from build123d import *
from build123d.topology import SkipClean

# Parameters (mm, degrees)
CIRPATTERN2_COUNT  = 6
SKETCH8_R          = 2.286
CUT_EXTRUDE1_DEPTH = 117.853803532


with BuildPart() as part:
    # Sketch3 → Revolve1 (revolve)
    with BuildSketch(Plane(origin=(0, 0, 0), x_dir=(0, 0, -1), z_dir=(1, 0, 0)), mode=Mode.PRIVATE) as revolve1_sk:
        with BuildLine():
            Line((0, 29.21), (0, 58.42))
            ThreePointArc((0, 58.42), (0.371974388, 59.318025612), (1.27, 59.69))
            Line((1.27, 59.69), (10.069743879, 59.69))
            ThreePointArc((10.069743879, 59.69), (12.499783674, 60.173364969), (14.559871939, 61.549871939))
            Line((14.559871939, 61.549871939), (21.000128061, 67.990128061))
            ThreePointArc((21.000128061, 67.990128061), (23.060216326, 69.366635031), (25.490256121, 69.85))
            Line((25.490256121, 69.85), (40.64, 69.85))
            Line((40.64, 69.85), (40.64, 77.47))
            Line((40.64, 77.47), (43.18, 77.47))
            Line((43.18, 77.47), (43.18, 67.31))
            Line((43.18, 67.31), (24.1935, 67.31))
            Line((24.1935, 67.31), (14.0335, 57.15))
            Line((14.0335, 57.15), (8.4455, 57.15))
            Line((8.4455, 57.15), (8.4455, 54.61))
            Line((8.4455, 54.61), (4.445, 54.61))
            ThreePointArc((4.445, 54.61), (3.546974388, 54.238025612), (3.175, 53.34))
            Line((3.175, 53.34), (3.175, 29.21))
            Line((3.175, 29.21), (0, 29.21))
        make_face()
    revolve(revolve1_sk.sketch.rotate(Axis((0, 0, 0), (0, 0, -1)), 90), axis=Axis((0, 0, 0), (0, 0, -1)))

    # Sketch7 → CSK for M4 Countersunk Flat Head Screw2 (revolve, cut)
    with BuildSketch(Plane(origin=(0, 35, -3.175), x_dir=(0, 1, 0), z_dir=(1, 0, 0))):
        Polygon((0, 0), (0, 4.526936393), (2.25, 3.175), (2.25, 2.45), (4.7, 0), align=None)
    csk_for_m4_countersunk_flat_head_screw2 = revolve(axis=Axis((0, 35, -9.525), (0, 0, 1)), mode=Mode.SUBTRACT)

    # CirPattern2: CSK for M4 Countersunk Flat Head Screw2 ×6 about axis
    cirpattern2_axis = Axis((0, 0, 0), (0, 0, 1))
    for i in range(1, CIRPATTERN2_COUNT):
        add(csk_for_m4_countersunk_flat_head_screw2.rotate(cirpattern2_axis, i * 360 / CIRPATTERN2_COUNT), mode=Mode.SUBTRACT)

    # Sketch8 → Cut-Extrude1 (cut, through all)
    with SkipClean():  # the faces are left unmerged after this step: merging them gives an invalid solid
        with BuildSketch(Plane.XY.offset(-40.64)):
            with BuildLine():
                ThreePointArc((77.47, 0), (75.984990618, 15.095764333), (71.586894261, 29.612792338))
                ThreePointArc((71.586894261, 29.612792338), (72.045629184, 26.639866522), (71.084638604, 23.789388889))
                Line((71.084638604, 23.789388889), (68.920030414, 20.36953457))
                ThreePointArc((68.920030414, 20.36953457), (68.026910163, 18.04667064), (68.095090227, 15.558958417))
                ThreePointArc((68.095090227, 15.558958417), (69.409886012, 7.828807306), (69.85, 0))
                ThreePointArc((69.85, 0), (69.409886012, -7.828807306), (68.095090227, -15.558958417))
                ThreePointArc((68.095090227, -15.558958417), (68.026910163, -18.04667064), (68.920030414, -20.36953457))
                Line((68.920030414, -20.36953457), (71.084638604, -23.789388889))
                ThreePointArc((71.084638604, -23.789388889), (72.045629184, -26.639866522), (71.586894261, -29.612792338))
                ThreePointArc((71.586894261, -29.612792338), (75.984990618, -15.095764333), (77.47, 0))
            make_face()
            with BuildLine():
                ThreePointArc((10.148016689, -76.802465177), (38.735, -67.090988031), (61.438877572, -47.189672839))
                ThreePointArc((61.438877572, -47.189672839), (59.093615754, -49.073411844), (56.14453442, -49.666408405))
                Line((56.14453442, -49.666408405), (52.100549608, -49.501729883))
                ThreePointArc((52.100549608, -49.501729883), (49.642330309, -49.889697022), (47.521998359, -51.192598801))
                ThreePointArc((47.521998359, -51.192598801), (41.484889014, -56.196320907), (34.925, -60.491874454))
                ThreePointArc((34.925, -60.491874454), (27.924996998, -64.025128213), (20.573091868, -66.751557218))
                ThreePointArc((20.573091868, -66.751557218), (18.384579854, -67.936367662), (16.819480806, -69.871264453))
                Line((16.819480806, -69.871264453), (14.940104183, -73.455797294))
                ThreePointArc((14.940104183, -73.455797294), (12.952013431, -75.713278366), (10.148016689, -76.802465177))
            make_face()
            with BuildLine():
                ThreePointArc((-56.14453442, -49.666408405), (-59.093615754, -49.073411844), (-61.438877572, -47.189672839))
                ThreePointArc((-61.438877572, -47.189672839), (-38.735, -67.090988031), (-10.148016689, -76.802465177))
                ThreePointArc((-10.148016689, -76.802465177), (-12.952013431, -75.713278366), (-14.940104183, -73.455797294))
                Line((-14.940104183, -73.455797294), (-16.819480806, -69.871264453))
                ThreePointArc((-16.819480806, -69.871264453), (-18.384579854, -67.936367662), (-20.573091868, -66.751557218))
                ThreePointArc((-20.573091868, -66.751557218), (-27.924996998, -64.025128213), (-34.925, -60.491874454))
                ThreePointArc((-34.925, -60.491874454), (-41.484889014, -56.196320907), (-47.521998359, -51.192598801))
                ThreePointArc((-47.521998359, -51.192598801), (-49.642330309, -49.889697022), (-52.100549608, -49.501729883))
                Line((-52.100549608, -49.501729883), (-56.14453442, -49.666408405))
            make_face()
            with BuildLine():
                ThreePointArc((-71.084638604, 23.789388889), (-72.045629184, 26.639866522), (-71.586894261, 29.612792338))
                ThreePointArc((-71.586894261, 29.612792338), (-77.47, 0), (-71.586894261, -29.612792338))
                ThreePointArc((-71.586894261, -29.612792338), (-72.045629184, -26.639866522), (-71.084638604, -23.789388889))
                Line((-71.084638604, -23.789388889), (-68.920030414, -20.36953457))
                ThreePointArc((-68.920030414, -20.36953457), (-68.026910163, -18.04667064), (-68.095090227, -15.558958417))
                ThreePointArc((-68.095090227, -15.558958417), (-69.409886012, -7.828807306), (-69.85, 0))
                ThreePointArc((-69.85, 0), (-69.409886012, 7.828807306), (-68.095090227, 15.558958417))
                ThreePointArc((-68.095090227, 15.558958417), (-68.026910163, 18.04667064), (-68.920030414, 20.36953457))
                Line((-68.920030414, 20.36953457), (-71.084638604, 23.789388889))
            make_face()
            with BuildLine():
                ThreePointArc((-14.940104183, 73.455797294), (-12.952013431, 75.713278366), (-10.148016689, 76.802465177))
                ThreePointArc((-10.148016689, 76.802465177), (-38.735, 67.090988031), (-61.438877572, 47.189672839))
                ThreePointArc((-61.438877572, 47.189672839), (-59.093615754, 49.073411844), (-56.14453442, 49.666408405))
                Line((-56.14453442, 49.666408405), (-52.100549608, 49.501729883))
                ThreePointArc((-52.100549608, 49.501729883), (-49.642330309, 49.889697022), (-47.521998359, 51.192598801))
                ThreePointArc((-47.521998359, 51.192598801), (-41.484889014, 56.196320907), (-34.925, 60.491874454))
                ThreePointArc((-34.925, 60.491874454), (-27.924996998, 64.025128213), (-20.573091868, 66.751557218))
                ThreePointArc((-20.573091868, 66.751557218), (-18.384579854, 67.936367662), (-16.819480806, 69.871264453))
                Line((-16.819480806, 69.871264453), (-14.940104183, 73.455797294))
            make_face()
            with BuildLine():
                ThreePointArc((10.148016689, 76.802465177), (12.952013431, 75.713278366), (14.940104183, 73.455797294))
                Line((14.940104183, 73.455797294), (16.819480806, 69.871264453))
                ThreePointArc((16.819480806, 69.871264453), (18.384579854, 67.936367662), (20.573091868, 66.751557218))
                ThreePointArc((20.573091868, 66.751557218), (27.924996998, 64.025128213), (34.925, 60.491874454))
                ThreePointArc((34.925, 60.491874454), (41.484889014, 56.196320907), (47.521998359, 51.192598801))
                ThreePointArc((47.521998359, 51.192598801), (49.642330309, 49.889697022), (52.100549608, 49.501729883))
                Line((52.100549608, 49.501729883), (56.14453442, 49.666408405))
                ThreePointArc((56.14453442, 49.666408405), (59.093615754, 49.073411844), (61.438877572, 47.189672839))
                ThreePointArc((61.438877572, 47.189672839), (38.735, 67.090988031), (10.148016689, 76.802465177))
            make_face()
            with Locations((0, 73.025)):
                Circle(SKETCH8_R)
            with Locations((63.241505111, 36.5125)):
                Circle(SKETCH8_R)
            with Locations((-63.241505111, 36.5125)):
                Circle(SKETCH8_R)
            with Locations((-63.241505111, -36.5125)):
                Circle(SKETCH8_R)
            with Locations((63.241505111, -36.5125)):
                Circle(SKETCH8_R)
            with Locations((0, -73.025)):
                Circle(SKETCH8_R)
        extrude(amount=-CUT_EXTRUDE1_DEPTH, mode=Mode.SUBTRACT)


solid = part.part
Geometry check sheet. Reference: the model listing, model coordinates, mm. A direction names the side the tool comes from. Round coordinates to 2 decimals unless told otherwise and drop trailing zeros. Write each loop counter-clockwise with the first axis right and the second up, starting at its lowest first coordinate (ties: lowest second). Pieces come first, ordered by that corner, then holes. Notation, with made-up numbers: (85, 2.25) -> (111, 2.25) arc R12 ccw to (111, 11.25) -> close; hole circle Ø7 at (13, 69.25). An arc over 180 degrees is marked (long way). One line per item, written item: value. Start each with the question number.
(1) Access from +Z, -Z, +X, -X, +Y, -Y to the whole of each face (thin tool, end or side, straight path). Record for faces 4 (the cylindrical face through (67.162, -38.612, -41.928)), 5 (the flat face through (60.8, -36.1, -40.64)), 6 (the flat face through (23, 23, -3.175)), 7 (the flat face through (60.8, 35.9, -40.64)), 8 (the cylindrical face through (12.917, 75.738, -41.892)).
(2) Go/stop test with flat-tipped pins: pin 1 Ø3.5 at (x, y) = (-30.31, 17.5) entering from +Z; pin 2 Ø10 at (x, y) = (-43.5, 6.5) entering from -Z (3 decimals); pin 3 Ø5 at (x, z) = (37.5, -30.5) entering from +Y; pin 4 Ø2 at (x, y) = (-39.5, 56) entering from +Z. Record where each tip stops, or that it passes through.
(3) Scan lines: line 1 (X direction, y = -2, z = -6); line 2 (Y direction, x = 0, z = -2) (3 decimals); line 3 (X direction, y = 17.5, z = -0.45). Record each from-to range of solid material in increasing order. Write a range as [from, to].
(4) Draft check along X on faces 1 (the cylindrical face through (-3.8, -28.96, -1.57)), 2 (the cylindrical face through (-67.162, 38.612, -41.928)), 3 (the flat face through (27, 12, 0)). Enter one of: +X half, -X half, draft (parallel to the pull), parting line (faces both ways), or undercut.
(5) Cross-section at B-B, the plane z = -38.5. Record the cut outline in (x, y).
(6) Cross-section at A-A, the plane x = 0. Give the number of separate pieces and of enclosed holes in the cut face, and give its area (3 significant figures).
Answer:
1. face 4: +Z, -Z, +X, -Y
1. face 5: +Z, +X, -Y
1. face 6: -Z
1. face 7: +Z, +X, +Y
1. face 8: +Z, -Z, +X, +Y
2. pin 1: through
2. pin 2: z = -3.175
2. pin 3: y = 60.45
2. pin 4: z = -20.54
3. line 1: [-59.66, -54.57], [54.57, 59.66]
3. line 2: [-59.69, -38.525], [-31.475, -29.21], [29.21, 31.475], [38.525, 59.69]
3. line 3: [-56.75, -32.56], [-28.06, -23.39], [23.39, 28.06], [32.56, 56.75]
4. face 1: undercut
4. face 2: -X half
4. face 3: draft
5. outline: circle Ø139.7 at (0, 0); hole circle Ø134.62 at (0, 0)
6. separate pieces: 6
6. enclosed holes: 0
6. area: 426 mm²
